For this review, take the finished solid that the model builds, in its own axes (mm). Coordinates: 2 decimals unless noted, no trailing zeros. Loops run counter-clockwise (first coordinate to the right, second up) from the corner with the lowest first, then second, coordinate; pieces in that order, holes last. Notation, with made-up numbers: M 83.25,-3 L 107.25,-3 A10 ccw 107.25,11 Z; hole C -37.75,9.25 d7. An arc over 180 degrees is marked long. Write each question's results on one line, items separated by ' | '. Start each with the question number.
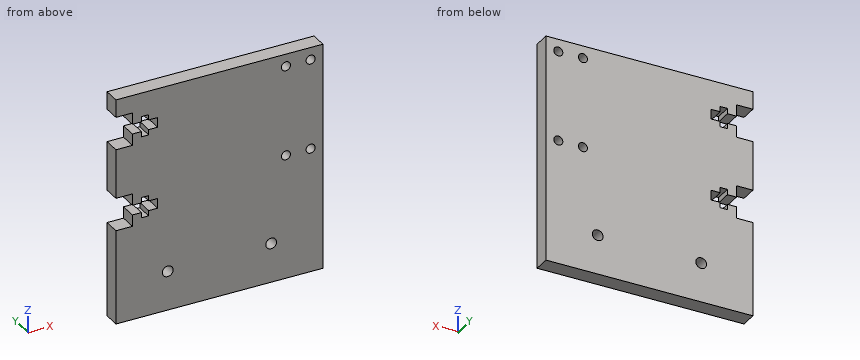
```python
from build123d import *

# Parameters (mm, degrees)
SKETCH1_W             = 80
SKETCH1_H             = 87.884
BOSS_EXTRUDE1_DEPTH   = 3.175
F_6_CLEARANCE_HOLE1_D = 3.5052
LPATTERN1_COUNT       = 2
LPATTERN1_PITCH       = 9.525
LPATTERN1_COUNT_DIR2  = 2
LPATTERN1_PITCH_DIR2  = 34.925
CUT_EXTRUDE1_REACH    = 61.76
LPATTERN3_COUNT       = 2
LPATTERN3_PITCH       = 31.75
SKETCH10_R            = 2.0828
CUT_EXTRUDE2_DEPTH    = 60.759701003


with BuildPart() as part:
    # Sketch1 → Boss-Extrude1 (new, symmetric)
    with BuildSketch(Plane(origin=(0, 0, 0), x_dir=(1, 0, 0), z_dir=(0, 1, 0))):
        Rectangle(SKETCH1_W, SKETCH1_H)
    extrude(amount=BOSS_EXTRUDE1_DEPTH, both=True)

    # #6 Clearance Hole1 (through all)
    with Locations(Plane(origin=(0, 3.175, 0), x_dir=(1, 0, 0), z_dir=(0, 1, 0))):
        with Locations((35.2375, -39.1795)):
            f_6_clearance_hole1 = Hole(F_6_CLEARANCE_HOLE1_D / 2)

    # LPattern1: 6 Clearance Hole1 2 × 2
    with Locations(*[(-i * LPATTERN1_PITCH, 0, -j * LPATTERN1_PITCH_DIR2) for i in range(LPATTERN1_COUNT) for j in range(LPATTERN1_COUNT_DIR2) if (i, j) != (0, 0)]):
        add(f_6_clearance_hole1, mode=Mode.SUBTRACT)

    # Sketch7 → Cut-Extrude1 (cut, up to next)
    with BuildSketch(Plane(origin=(0, 3.175, 0), x_dir=(1, 0, 0), z_dir=(0, 1, 0)), mode=Mode.PRIVATE) as cut_extrude1_sk1:
        Polygon((-40, 7.366), (-40, -5.334), (-33.65, -5.334), (-33.65, -0.88265), (-30.1495625, -0.88265), (-30.1495625, -2.95275), (-27.3714375, -2.95275), (-27.3714375, -0.88265), (-23.871, -0.88265), (-23.871, 2.91465), (-27.3714375, 2.91465), (-27.3714375, 4.98475), (-30.1495625, 4.98475), (-30.1495625, 2.91465), (-33.65, 2.91465), (-33.65, 7.366), align=None)
    cut_extrude1_tool1 = extrude(cut_extrude1_sk1.sketch, amount=-CUT_EXTRUDE1_REACH, mode=Mode.PRIVATE) & part.part
    cut_extrude1 = cut_extrude1_tool1.solids().sort_by_distance((-33.791113, 3.175, -1.016))[0]
    add(cut_extrude1, mode=Mode.SUBTRACT)

    # LPattern3: Cut-Extrude1 ×2
    with Locations(*[(0, 0, i * LPATTERN3_PITCH) for i in range(1, LPATTERN3_COUNT)]):
        add(cut_extrude1, mode=Mode.SUBTRACT)

    # Sketch10 → Cut-Extrude2 (cut, through all)
    with BuildSketch(Plane(origin=(0, 3.175, 0), x_dir=(1, 0, 0), z_dir=(0, 1, 0))):
        with Locations(Location((20, 28.733, 0), (0, 0, 270))):
            Circle(SKETCH10_R)
        with Locations(Location((-20, 28.733, 0), (0, 0, 270))):
            Circle(SKETCH10_R)
    extrude(amount=-CUT_EXTRUDE2_DEPTH, mode=Mode.SUBTRACT)


solid = part.part
```
Q1. Take a section at B-B, the plane z = 31.5. Give the boundary of the cut face in (x, y) (3 decimals).
Q2. To check wall thickness, follow line 1 along X through (y, z) = (2, 33); line 2 along X through (y, z) = (1.75, 3.5); line 3 along Z through (x, y) = (36.5, -1.75). State the ranges of each line that lie inside material, in increasing order.
Q3. Take a section at C-C, the plane y = 0.5. Give the number of separate pieces and of enclosed holes in the cut face, then the cut area to 3 significant figures.
Q4. Insertion check: P1, Ø1.3, axis at y = -1, z = -5.5, coming from the -X side. The pin has a flat end and moves straight along its axis. Give the tip position at first contact, or say it passes through.
Q5. Take a section at A-A, the plane x = -20. Give the boundary of the cut face in (y, z) (3 decimals).
Results:
1) outline: M -23.871,-3.175 L 40,-3.175 L 40,3.175 L -23.871,3.175 Z
2) line 1: -33.65 to -30.15, -27.37 to 40 | line 2: -33.65 to 24.13, 27.29 to 33.66, 36.82 to 40 | line 3: -43.94 to 3.04, 5.47 to 37.96, 40.4 to 43.94
3) separate pieces: 1 | enclosed holes: 6 | area: 6,710 mm^2
4) P1: x = -33.65
5) outline: M -3.175,-43.942 L 3.175,-43.942 L 3.175,-30.816 L -3.175,-30.816 Z; M -3.175,-26.65 L 3.175,-26.65 L 3.175,43.942 L -3.175,43.942 Z
